Input: part model. Units: mm. Frame: model coordinates. A direction names the side the tool comes from. Round coordinates to 2 decimals unless told otherwise and drop trailing zeros. Loops run counter-clockwise (first coordinate to the right, second up) from the corner with the lowest first, then second, coordinate; pieces in that order, holes last. Notation, with made-up numbers: (-21.5, 60.25) -> (21.5, 60.25) arc R23 cw to (21.5, 69.25) -> close; hole circle Ø9 at (23, -7). An arc over 180 degrees is marked (long way). Answer as a JSON object with one key per item and string values. Group by question number.
Item 1: Set-up query: faces 1 (the flat face through (-121, 50.8, 3)), 2 (the flat face through (-28.575, 9, 3)), 3 (the flat face through (121, -25.4, 3)). Return all of +Z, -Z, +X, -X, +Y, -Y with unobstructed straight access to the full face (end or side cutting, diameter ignored); none if empty.
Item 2: Draft query along X for faces 4 (the flat face through (57, 6.35, 3)), 5 (the flat face through (117.475, -32, 3)), 6 (the flat face through (-117.475, -32, 3)). Return one class per face: released by +X, released by -X, zero draft, split by the parting line, or undercut.
Item 3: Material intervals for line 1 (Y direction, x = 94, z = 0.75); line 2 (X direction, y = 40, z = 2.5) (3 decimals), sorted ascending. Write a range as [from, to].
Item 4: Pin query (flat end, axial travel): pin 1 (1.9 mm diameter, centred on y = 44.5, z = 2, fed in from +X) (3 decimals); pin 2 (6 mm diameter, centred on x = -90.5, y = 49.5, fed in from -Z). Return the tip coordinate at first contact, or that it passes through.
Item 5: Section query A-A on x = -20. Return loops of the section in (y, z), and give its area (3 significant figures).
Item 6: Section query B-B on z = 5. Count the separate pieces of the cut face and the enclosed holes in it, and give its area (3 significant figures).
Item 7: Section query C-C on y = 48. Return loops of the section in (x, z) (3 decimals).
from build123d import *

# Parameters (mm, degrees)
ESQUISSE1_W                     = 247.65
ESQUISSE1_H                     = 127
BOSS_EXTRU_1_DEPTH              = 6.35
ESQUISSE2_W                     = 19.05
ESQUISSE2_H                     = 6.35
ENL_V_MAT_EXTRU_1_DEPTH         = 6.35
R_P_TITION_LIN_AIRE1_COUNT      = 6
R_P_TITION_LIN_AIRE1_PITCH      = 38.1
R_P_TITION_LIN_AIRE1_COUNT_DIR2 = 2
R_P_TITION_LIN_AIRE1_PITCH_DIR2 = 57.15
ESQUISSE3_W                     = 6.35
ESQUISSE3_H                     = 12.7
ENL_V_MAT_EXTRU_2_DEPTH         = 6.35
R_P_TITION_LIN_AIRE2_COUNT      = 4
R_P_TITION_LIN_AIRE2_PITCH      = 25.4
R_P_TITION_LIN_AIRE2_COUNT_DIR2 = 2
R_P_TITION_LIN_AIRE2_PITCH_DIR2 = 241.3


with BuildPart() as part:
    # Esquisse1 → Boss.-Extru.1 (new body)
    with BuildSketch(Plane.XY):
        Rectangle(ESQUISSE1_W, ESQUISSE1_H)
    extrude(amount=BOSS_EXTRU_1_DEPTH)

    # Esquisse2 → Enlèv. mat.-Extru.1 (cut)
    with BuildSketch(Plane.XY.offset(6.35)):
        with Locations((-95.25, 9.525)):
            Rectangle(ESQUISSE2_W, ESQUISSE2_H)
    enl_v_mat_extru_1 = extrude(amount=-ENL_V_MAT_EXTRU_1_DEPTH, mode=Mode.SUBTRACT)

    # Répétition linéaire1: Enl_v. mat.-Extru.1 6 × 2
    with Locations(*[(i * R_P_TITION_LIN_AIRE1_PITCH, j * R_P_TITION_LIN_AIRE1_PITCH_DIR2, 0) for i in range(R_P_TITION_LIN_AIRE1_COUNT) for j in range(R_P_TITION_LIN_AIRE1_COUNT_DIR2) if (i, j) != (0, 0)]):
        add(enl_v_mat_extru_1, mode=Mode.SUBTRACT)

    # Esquisse3 → Enlèv. mat.-Extru.2 (cut)
    with BuildSketch(Plane.XY.offset(6.35)):
        with Locations((-120.65, 44.45)):
            Rectangle(ESQUISSE3_W, ESQUISSE3_H)
    enl_v_mat_extru_2 = extrude(amount=-ENL_V_MAT_EXTRU_2_DEPTH, mode=Mode.SUBTRACT)

    # Répétition linéaire2: Enl_v. mat.-Extru.2 4 × 2
    with Locations(*[(j * R_P_TITION_LIN_AIRE2_PITCH_DIR2, -i * R_P_TITION_LIN_AIRE2_PITCH, 0) for i in range(R_P_TITION_LIN_AIRE2_COUNT) for j in range(R_P_TITION_LIN_AIRE2_COUNT_DIR2) if (i, j) != (0, 0)]):
        add(enl_v_mat_extru_2, mode=Mode.SUBTRACT)


solid = part.part
Solved:
{
 "1": {"face 1": "+Z, -Z, -X", "face 2": "+Z, -Z", "face 3": "+Z, -Z, +X"},
 "2": {"face 4": "undercut", "face 5": "released by +X", "face 6": "released by -X"},
 "3": {"line 1": "[-63.5, 6.35], [12.7, 63.5]", "line 2": "[-117.475, 117.475]"},
 "4": {"pin 1": "x = 117.475", "pin 2": "z = 0"},
 "5": {"outline": "(-63.5, 0) -> (6.35, 0) -> (6.35, 6.35) -> (-63.5, 6.35) -> close; (12.7, 0) -> (63.5, 0) -> (63.5, 6.35) -> (12.7, 6.35) -> close", "area": "766 mm²"},
 "6": {"separate pieces": "1", "enclosed holes": "6", "area": "30,100 mm²"},
 "7": {"outline": "(-117.475, 0) -> (117.475, 0) -> (117.475, 6.35) -> (-117.475, 6.35) -> close"}
}
